The model under review builds one solid part; all positions refer to its coordinate system, in mm. A direction names the side the tool comes from. Coordinates: 2 decimals unless noted, no trailing zeros. Write each loop counter-clockwise with the first axis right and the second up, starting at its lowest first coordinate (ties: lowest second). Pieces come first, ordered by that corner, then holes. Notation, with made-up numbers: M 65.25,43 L 91.25,43 A14 ccw 91.25,62 Z; hole C 25,77.5 d8. An arc over 180 degrees is marked long. Answer as a JSON object with one key per item and string values.
```python
from build123d import *

# Parameters (mm, degrees)
SKETCH1_W           = 20
SKETCH1_H           = 50
BOSS_EXTRUDE1_DEPTH = 4
SKETCH2_W           = 40
SKETCH2_H           = 20
BOSS_EXTRUDE2_DEPTH = 4
SKETCH3_R           = 1.2
SKETCH3_R_2         = 2
CUT_EXTRUDE1_DEPTH  = 4
SKETCH4_W           = 40
SKETCH4_H           = 20
BOSS_EXTRUDE3_DEPTH = 4
SKETCH5_R           = 5.2
CUT_EXTRUDE2_DEPTH  = 4
CHAMFER1_SIZE       = 1
SKETCH6_R           = 2
SKETCH6_R_2         = 1.2
CUT_EXTRUDE3_DEPTH  = 10


with BuildPart() as part:
    # Sketch1 → Boss-Extrude1 (new body)
    with BuildSketch(Plane(origin=(0, 0, 0), x_dir=(0, 0, -1), z_dir=(1, 0, 0))):
        Rectangle(SKETCH1_W, SKETCH1_H)
    extrude(amount=BOSS_EXTRUDE1_DEPTH)

    # Sketch2 → Boss-Extrude2 (add)
    with BuildSketch(Plane(origin=(0, 25, 0), x_dir=(1, 0, 0), z_dir=(0, 1, 0))):
        with Locations((20, 0)):
            Rectangle(SKETCH2_W, SKETCH2_H)
    extrude(amount=BOSS_EXTRUDE2_DEPTH)

    # Sketch3 → Cut-Extrude1 (cut)
    with BuildSketch(Plane(origin=(0, 29, 0), x_dir=(1, 0, 0), z_dir=(0, 1, 0))):
        with Locations(Location((33, 0, 0), (0, 0, 270))):
            Circle(SKETCH3_R)
        with Locations(Location((26, 0, 0), (0, 0, 270))):
            Circle(SKETCH3_R_2)
        with Locations(Location((26, -7, 0), (0, 0, 270))):
            Circle(SKETCH3_R)
        with Locations(Location((19, 0, 0), (0, 0, 270))):
            Circle(SKETCH3_R)
        with Locations(Location((26, 7, 0), (0, 0, 270))):
            Circle(SKETCH3_R)
    extrude(amount=-CUT_EXTRUDE1_DEPTH, mode=Mode.SUBTRACT)

    # Sketch4 → Boss-Extrude3 (add)
    with BuildSketch(Plane.XZ.offset(25)):
        with Locations((20, 0)):
            Rectangle(SKETCH4_W, SKETCH4_H)
    extrude(amount=BOSS_EXTRUDE3_DEPTH)

    # Sketch5 → Cut-Extrude2 (cut)
    with BuildSketch(Plane.XZ.offset(29)):
        with Locations(Location((26, 0, 0), (0, 0, 270))):
            Circle(SKETCH5_R)
    extrude(amount=-CUT_EXTRUDE2_DEPTH, mode=Mode.SUBTRACT)

    # Chamfer1
    chamfer1_edges = [part.edges().sort_by_distance(p)[0] for p in [
        (4, 0, 10),
        (4, -25, 0),
        (22, 25, 10),
        (40, 25, 0),
        (40, 27, 10),
        (22, 25, -10),
        (40, 27, -10),
        (0, 29, 0),
        (20, 29, 10),
        (40, 29, 0),
        (20, 29, -10),
        (4, 0, -10),
        (0, 0, 10),
        (22, -25, -10),
        (40, -25, 0),
        (40, -27, -10),
        (22, -25, 10),
        (40, -27, 10),
        (0, -29, 0),
        (20, -29, -10),
        (40, -29, 0),
        (20, -29, 10),
        (0, 0, -10),
        (4, 25, 0),
    ]]
    chamfer(chamfer1_edges, length=CHAMFER1_SIZE)

    # Sketch6 → Cut-Extrude3 (cut)
    with BuildSketch(Plane.ZY):
        Circle(SKETCH6_R)
        with Locations((7, 0)):
            Circle(SKETCH6_R_2)
        with Locations((0, -7)):
            Circle(SKETCH6_R_2)
        with Locations((-7, 0)):
            Circle(SKETCH6_R_2)
        with Locations((0, 7)):
            Circle(SKETCH6_R_2)
    extrude(amount=-CUT_EXTRUDE3_DEPTH, mode=Mode.SUBTRACT)


solid = part.part
```
(1) For faces 1 (the face through (4.2, -24.8, -9.6)), 2 (the face through (24.83, 27.03, 6.74)), 3 (the face through (4, 0.34, 2.13)), 4 (the face through (20.924, -27.028, 1.127)), list the 3-axis set-ups (+Z, -Z, +X, -X, +Y, -Y) from which the entire face can be reached by the end or side of a thin tool; tool diameter is ignored.
Results list:
{"face 1": "-Z, +X", "face 2": "+Y", "face 3": "+Z, -Z, +X", "face 4": "-Y"}
(2) For pin 1 Ø8 at (x, y) = (5, 16) entering from -Z; pin 2 Ø2 at (y, z) = (7, 2) entering from +X; pin 3 Ø3 at (y, z) = (0, 0) entering from +X; pin 4 Ø5.5 at (x, z) = (25.5, 0.5) entering from -Y, all flat-tipped, find the tip position at first contact; note any pin that passes through.
Results list:
{"pin 1": "z = -10", "pin 2": "x = 4", "pin 3": "through", "pin 4": "y = 25"}
(3) Add section C-C on x = 26. Count the separate pieces of the cut face and the enclosed holes in it, and give its area (3 significant figures).
Results list:
{"separate pieces": "6", "enclosed holes": "0", "area": "79.2 mm²"}
(4) Add section A-A on x = 33. Give the boundary of the cut face in (y, z).
Results list:
{"outline": "M -29,-9 L -28,-10 L -26,-10 L -25,-9 L -25,9 L -26,10 L -28,10 L -29,9 Z; M 25,-9 L 26,-10 L 28,-10 L 29,-9 L 29,-1.2 L 25,-1.2 Z; M 25,1.2 L 29,1.2 L 29,9 L 28,10 L 26,10 L 25,9 Z"}
(5) Draft analysis for pull direction Z (two halves, no side actions). For faces 5 (the face through (40, -27, 0)), 6 (the face through (34.19, 27.03, -0.16)), 7 (the face through (4.2, 24.8, -9.6)), 8 (the face through (4.2, 24.8, 9.6)), state which applies: released by +Z, released by -Z, zero draft, split by the parting line, or undercut.
Results list:
{"face 5": "zero draft", "face 6": "undercut", "face 7": "released by -Z", "face 8": "released by +Z"}
(6) Wall thickness on line 1 along Y through (x, z) = (10, 7.5); line 2 along X through (y, z) = (26.7, 0); line 3 along X through (y, z) = (27.05, 7): over which ranges is each line inside the solid? List them lowest first. Write a range as from..to.
Results list:
{"line 1": "-29..-25, 25..29", "line 2": "0..17.8, 20.2..24, 28..31.8, 34.2..40", "line 3": "0..24.8, 27.2..40"}
(7) Add section D-D on y = 0. Give the boundary of the cut face in (x, z).
Results list:
{"outline": "M 0,-9 L 1,-10 L 3,-10 L 4,-9 L 4,-8.2 L 0,-8.2 Z; M 0,-5.8 L 4,-5.8 L 4,-2 L 0,-2 Z; M 0,2 L 4,2 L 4,5.8 L 0,5.8 Z; M 0,8.2 L 4,8.2 L 4,9 L 3,10 L 1,10 L 0,9 Z"}
(8) Add section B-B on y = 7. Give the boundary of the cut face in (x, z).
Results list:
{"outline": "M 0,-9 L 1,-10 L 3,-10 L 4,-9 L 4,-1.2 L 0,-1.2 Z; M 0,1.2 L 4,1.2 L 4,9 L 3,10 L 1,10 L 0,9 Z"}
